from build123d import *

# Parameters (mm, degrees)
F0_R     = 1.5
F0_R_2   = 2
F1_DEPTH = 1.5
F3_DEPTH = 36
F4_W     = 13.25
F4_H     = 3.5
F5_DEPTH = 25
F6_DEPTH = 25
F7_DEPTH = 1.5
F8_R     = 3.5


with BuildPart() as f1:
    # F0 (on Top) → F1 (new body)
    with BuildSketch(Plane.XY):
        Polygon((-4.012614, -5.998938), (-5.462614, -5.998938), (-5.462614, -11.098938), (-5.462614, -36.898938), (-5.462614, -41.998938), (-4.012614, -41.998938), (29.087386, -41.998938), (30.537386, -41.998938), (30.537386, -36.898938), (30.537386, -11.098938), (30.537386, -5.998938), (29.087386, -5.998938), align=None)
        with Locations((-2.712614, -39.248938)):
            Circle(F0_R, mode=Mode.SUBTRACT)
        with Locations((27.787386, -39.248938)):
            Circle(F0_R, mode=Mode.SUBTRACT)
        with Locations((-2.712614, -8.748938)):
            Circle(F0_R_2, mode=Mode.SUBTRACT)
        with Locations((27.787386, -8.748938)):
            Circle(F0_R_2, mode=Mode.SUBTRACT)
    extrude(amount=F1_DEPTH)

    # F2 (on face) → F3 (join)
    with BuildSketch(Plane(origin=(-5.462614, 0, 0), x_dir=(0, -1, 0), z_dir=(-1, 0, 0))):
        Polygon((28.094722, 0), (5.998938, 0), (5.998938, -10.303433), align=None)
    extrude(amount=-F3_DEPTH)

    # F4 (on face) → F5 (cut)
    with BuildSketch(Plane(origin=(0, -5.998938, 0), x_dir=(-1, 0, 0), z_dir=(0, 1, 0))):
        with Locations((-7.778386, -1.75)):
            Rectangle(F4_W, F4_H)
    extrude(amount=-F5_DEPTH, mode=Mode.SUBTRACT)

    # F0 (on Top) → F6 (cut)
    with BuildSketch(Plane.XY):
        with Locations((27.787386, -8.748938)):
            Circle(F0_R_2)
        with Locations((27.787386, -8.748938)):
            Circle(F0_R, mode=Mode.SUBTRACT)
        with Locations((-2.712614, -8.748938)):
            Circle(F0_R_2)
        with Locations((-2.712614, -8.748938)):
            Circle(F0_R, mode=Mode.SUBTRACT)
        with Locations((-2.712614, -8.748938)):
            Circle(F0_R)
        with Locations((27.787386, -8.748938)):
            Circle(F0_R)
    extrude(amount=-F6_DEPTH, mode=Mode.SUBTRACT)

    # F0 (on Top) → F7 (join)
    with BuildSketch(Plane.XY):
        with Locations((27.787386, -8.748938)):
            Circle(F0_R_2)
        with Locations((27.787386, -8.748938)):
            Circle(F0_R, mode=Mode.SUBTRACT)
        with Locations((-2.712614, -8.748938)):
            Circle(F0_R_2)
        with Locations((-2.712614, -8.748938)):
            Circle(F0_R, mode=Mode.SUBTRACT)
    extrude(amount=F7_DEPTH)

    # F8
    f8_edges = [f1.edges().sort_by_distance(p)[0] for p in [
        (-5.462614, -5.998938, -4.401717),
        (-5.462614, -41.998938, 0.75),
        (30.537386, -5.998938, -4.401717),
        (30.537386, -41.998938, 0.75),
    ]]
    fillet(f8_edges, radius=F8_R)


solid = f1.part
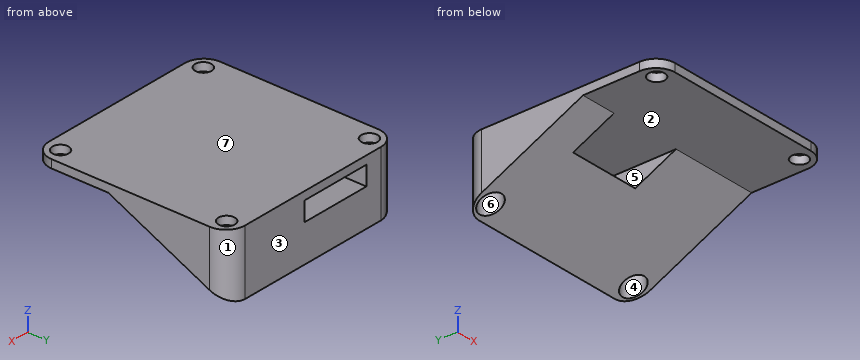
Input: part model. Units: mm. Frame: model coordinates. Face numbers are marked on the shaded views. A direction names the side the tool comes from. Coordinates: 2 decimals unless noted, no trailing zeros. Loops run counter-clockwise (first coordinate to the right, second up) from the corner with the lowest first, then second, coordinate; pieces in that order, holes last. Notation, with made-up numbers: (39, 15.25) -> (61, 15.25) arc R31 cw to (61, 45.25) -> close; hole circle Ø3 at (-15, 18.5). An arc over 180 degrees is marked (long way). Write item = value, one per line. Start each with the question number.
Item 1: Cut plane B-B, the plane z = -0.5. Return loops of the section in (x, y), plus the area to 3 significant figures.
Item 2: Reachability of the marked faces 5, 6 and 7 from +Z, -Z, +X, -X, +Y, -Y: full face, straight path, thin tool, end or side. Return the list, or none.
Item 3: Cut plane D-D, the plane y = -12.5. Return loops of the section in (x, z).
Item 4: Material intervals for line 1 (X direction, y = -24.5, z = -1.5); line 2 (Z direction, x = 10, y = -30.5); line 3 (Y direction, x = -3, z = -1.75), sorted ascending.
Item 5: Mould query, pull axis X, two halves, no side actions, for the marked faces 1, 2, 3 and 4. Classes: pulls with the +X half, pulls with the -X half, needs draft (parallel to the pull), parting line crosses it, or undercut.
Item 6: First-contact query: P1, Ø1, axis at x = 3, y = -36, coming from the -Z side; P2, Ø5, axis at x = 27.79, y = -8.75, coming from the -Z side; P3, Ø3.5, axis at x = -2.71, y = -8.75, coming from the +Z side; P4, Ø1.5, axis at x = 13, y = -17, coming from the -Z side. Flat tips, straight axial feed; report the tip coordinate or a pass-through.
Item 7: Cut plane C-C, the plane y = -40. Return loops of the section in (x, z).
Item 8: Cut plane A-A, the plane x = 2. Return loops of the section in (y, z).
Ans:
q1.outline = (-5.46, -27.02) -> (1.15, -27.02) -> (1.15, -6) -> (-1.96, -6) arc R3.5 ccw to (-5.46, -9.5) -> close; (14.4, -27.02) -> (30.54, -27.02) -> (30.54, -9.5) arc R3.5 ccw to (27.04, -6) -> (14.4, -6) -> close; hole circle Ø4 at (-2.71, -8.75); hole circle Ø4 at (27.79, -8.75)
q1.area = 448 mm²
q2.face_5 = +Y, -Y
q2.face_6 = -Z
q2.face_7 = +Z, +X, -X, +Y, -Y
q3.outline = (-5.46, -7.27) -> (30.54, -7.27) -> (30.54, 1.5) -> (-5.46, 1.5) -> close; hole (1.15, -3.5) -> (14.4, -3.5) -> (14.4, 0) -> (1.15, 0) -> close
q4.line_1 = -5.46 to 1.15, 14.4 to 30.54
q4.line_2 = 0 to 1.5
q4.line_3 = -24.34 to -10.73, -6.77 to -6.16
q5.face_1 = pulls with the +X half
q5.face_2 = undercut
q5.face_3 = needs draft
q5.face_4 = undercut
q6.P1 = 0
q6.P2 = -10.19
q6.P3 = 1.5
q6.P4 = -5.52
q7.outline = (-5.12, 0) -> (-4.01, 0) -> (-4.01, 1.5) -> (-5.12, 1.5) -> close; (-1.41, 0) -> (26.49, 0) -> (26.49, 1.5) -> (-1.41, 1.5) -> close; (29.09, 0) -> (30.2, 0) -> (30.2, 1.5) -> (29.09, 1.5) -> close
q8.outline = (-42, 0) -> (-6, 0) -> (-6, 1.5) -> (-42, 1.5) -> close; (-20.59, -3.5) -> (-6, -10.3) -> (-6, -3.5) -> close
